from build123d import *

# Parameters (mm, degrees)
F1_DEPTH = 25.4
F4_DEPTH = 25.4


with BuildPart() as f1:
    # F0 (on Front) → F1 (new body)
    with BuildSketch(Plane.XZ):
        Polygon((-29.4040627778, -34.6658416092), (-13.9282392338, -34.6658416092), (-13.9282392338, -54.4748939574), (0, -54.4748939574), (0, -34.0468101203), (12.9996910691, -34.0468101203), (0, -9.9045261741), (19.4995384663, -10.8330762014), (0, 19.4995366037), (12.9996910691, 19.4995366037), (-6.4998446032, 39.9276204407), (-25.3803487867, 19.8090523481), (-8.9759770781, 19.8090523481), (-34.6658416092, -9.9045261741), (-13.9282392338, -10.8330762014), align=None)
        Polygon((-20.9672786295, 22.1136379987), (-11.3465078175, 31.0843549669), (-6.3364817826, 36.2658323126), (6.7840320989, 22.5205328315), (-2.7060393941, 22.5205328315), (-2.7060393941, 17.6217724478), (12.9996910691, -6.8093617447), (-2.3284680181, -6.8093617447), (-2.3284680181, -12.9201814463), (8.0474307761, -32.1897082031), (-3.9969988042, -32.1897082031), (-3.9969988042, -51.0926617871), (-11.4108609159, -50.7606975734), (-11.4108609159, -31.906359816), (-23.4664510936, -31.3665568829), (-11.4108609159, -13.363099657), (-11.4108609159, -7.944371215), (-29.4040627778, -7.1387048811), (-7.8362263739, 19.4995366037), (-7.8362263739, 22.1136379987), align=None, mode=Mode.SUBTRACT)
    extrude(amount=F1_DEPTH)


with BuildPart() as f4:
    # F3 (on Front) → F4 (new body)
    with BuildSketch(Plane.XZ):
        Polygon((-24.4517996907, -40.5466556549), (-6.1903311871, -40.5466556549), (-6.1903311871, -56.3319921494), (5.2617802285, -56.3319921494), (5.2617802285, -41.784722358), (23.8327626139, -41.784722358), (5.2617802285, -9.2854928225), (27.8564821929, -9.2854928225), (5.2617802285, 19.1900189966), (23.8327626139, 19.1900189966), (0, 47.3560169339), (-24.4517996907, 19.1900189966), (-6.1903311871, 19.4995366037), (-24.4517996907, -10.8330762014), (-6.1903311871, -10.8330762014), align=None)
        Polygon((-17.1195007861, 21.893909201), (0, 43.7848083675), (15.8973690122, 21.893909201), (3.0488721095, 21.893909201), (3.0488721095, 14.5096303895), (20.8655081271, -6.5463982989), (3.0488721095, -6.5463982989), (3.0488721095, -13.4936347604), (15.8973690122, -36.6372689605), (17.5805799663, -40.379870683), (3.4944114741, -40.379870683), (2.7118462604, -54.1725791991), (-4.5268801041, -54.1725791991), (-4.5268801041, -38.5212786496), (-17.1195007861, -36.6372689605), (-3.9520426653, -13.4936347604), (-3.9520426653, -9.2854928225), (-20.0821794569, -9.2854928225), (-3.9520426653, 17.9436709732), (-3.9520426653, 21.893909201), align=None, mode=Mode.SUBTRACT)
    extrude(amount=F4_DEPTH)


solid = f4.part
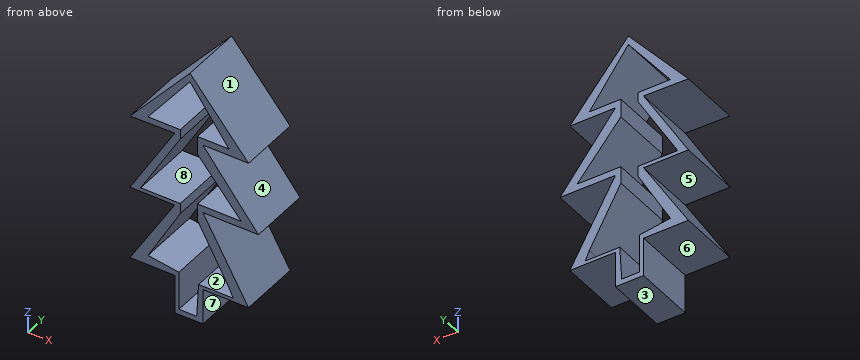
For this review, take the finished solid that the model builds, in its own axes (mm). Face numbers are marked on the shaded views. A direction names the side the tool comes from. Coordinates: 2 decimals unless noted, no trailing zeros. Order: outer loops, then holes, each group sorted by start corner. A loop starts at its lowest first (then second) coordinate and runs counter-clockwise, first axis right, second up. Notation, with made-up numbers: (59.5, -35) -> (71.5, -35) arc R11 cw to (71.5, -31) -> close; hole circle Ø11 at (-7.5, -13.5). An arc over 180 degrees is marked (long way). Return JSON: item names as keys, results as strings.
1. We need section A-A on z = -45.5. Write out the cut boundary in (x, y).
Answer block:
{"outline": "(-6.19, -25.4) -> (-4.53, -25.4) -> (-4.53, 0) -> (-6.19, 0) -> close; (3.2, -25.4) -> (5.26, -25.4) -> (5.26, 0) -> (3.2, 0) -> close"}
2. We need section B-B on x = 13. Write out the cut boundary in (y, z), and give its area (3 significant figures).
Answer block:
{"outline": "(-25.4, -41.78) -> (0, -41.78) -> (0, -40.38) -> (-25.4, -40.38) -> close; (-25.4, -31.42) -> (0, -31.42) -> (0, -22.83) -> (-25.4, -22.83) -> close; (-25.4, -9.29) -> (0, -9.29) -> (0, -6.55) -> (-25.4, -6.55) -> close; (-25.4, 2.75) -> (0, 2.75) -> (0, 9.44) -> (-25.4, 9.44) -> close; (-25.4, 19.19) -> (0, 19.19) -> (0, 21.89) -> (-25.4, 21.89) -> close; (-25.4, 25.88) -> (0, 25.88) -> (0, 31.99) -> (-25.4, 31.99) -> close", "area": "717 mm²"}
3. We need section D-D on x = -9. Write out the cut boundary in (y, z).
Answer block:
{"outline": "(-25.4, -40.55) -> (0, -40.55) -> (0, -37.85) -> (-25.4, -37.85) -> close; (-25.4, -22.37) -> (0, -22.37) -> (0, -15.4) -> (-25.4, -15.4) -> close; (-25.4, -10.83) -> (0, -10.83) -> (0, -9.29) -> (-25.4, -9.29) -> close; (-25.4, 9.42) -> (0, 9.42) -> (0, 14.83) -> (-25.4, 14.83) -> close; (-25.4, 19.45) -> (0, 19.45) -> (0, 21.89) -> (-25.4, 21.89) -> close; (-25.4, 32.28) -> (0, 32.28) -> (0, 36.99) -> (-25.4, 36.99) -> close"}
4. For pin 1 Ø14.5 at (x, y) = (-10, -19) entering from +Z; pin 2 Ø5 at (y, z) = (-21.5, -25) entering from +X; pin 3 Ø1.5 at (x, y) = (-2.5, -7.5) entering from +Z; pin 4 Ø12 at (x, z) = (12, -12.5) entering from +Y, all flat-tipped, find the tip position at first contact; note any pin that passes through.
Answer block:
{"pin 1": "z = 44.19", "pin 2": "x = 15.67", "pin 3": "z = 45.34", "pin 4": "y = 0"}
5. Machinability: for the marked faces 4, 5, 6, 7 and 8, which of the approach directions +Z, -Z, +X, -X, +Y, -Y give a long, thin tool a straight path to every point of the face, cutting with its end or side? Answer none if there is none.
Answer block:
{"face 4": "+X, +Y, -Y", "face 5": "-X, +Y, -Y", "face 6": "-Z, -X, +Y, -Y", "face 7": "-Z, +X, +Y, -Y", "face 8": "+Y, -Y"}
6. The part is to be moulded in two halves that separate along Z. For the marked faces 1, 2 and 3, say which applies: +Z half, -Z half, draft (parallel to the pull), parting line (faces both ways), or undercut.
Answer block:
{"face 1": "+Z half", "face 2": "undercut", "face 3": "-Z half"}
7. For line 1 (Z direction, x = -15, y = -13.25); line 2 (Z direction, x = 15.5, y = -8.25); line 3 (Z direction, x = 18, y = -8.25), list the stretches that pass through material, from the lowest coordinate up. Write a range as from..to.
Answer block:
{"line 1": "-40.55..-36.95, -32.91..-25.17, -10.83..-9.29, -0.71..4.87, 19.35..21.89, 24.6..30.08", "line 2": "-41.78..-40.38, -35.92..-27.2, -9.29..-6.55, -0.21..6.29, 19.19..21.89, 22.44..29.04", "line 3": "-41.78..-31.58, -9.29..-6.55, -3.16..3.14, 19.19..26.08"}
8. We need section C-C on z = 7.5. Write out the cut boundary in (x, y).
Answer block:
{"outline": "(-13.41, -25.4) -> (-10.14, -25.4) -> (-10.14, 0) -> (-13.41, 0) -> close; (8.98, -25.4) -> (14.54, -25.4) -> (14.54, 0) -> (8.98, 0) -> close"}
